Could you check a few things on this drawing? It's one solid part, dimensions in mm from its lowest x, y, z. Give positions to 0.01 mm unless a question says otherwise; leave off trailing zeros. Order: outer loops, then holes, each group sorted by start corner. A loop starts at its lowest first (then second) coordinate and runs counter-clockwise, first axis right, second up. Notation, with made-up numbers: M -16.5,40 L -4.5,40 A18 ccw -4.5,67 Z; hole C 4,22.5 d5. An arc over 180 degrees is marked long. Use CSV: the item, a comma, the result in double quotes. Start each with the question number.
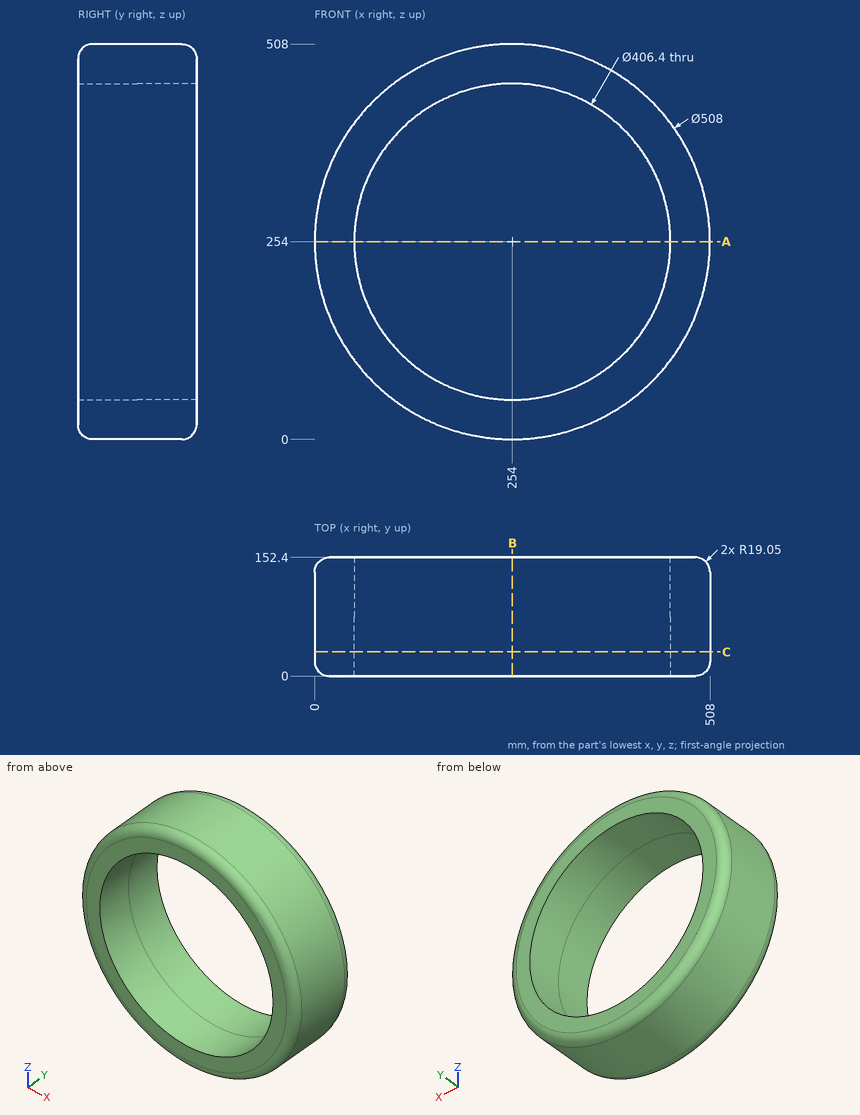
Q1. For P1, Ø1.5, axis at x = 429.5, y = 68, coming from the -Z side; P2, Ø12, axis at x = 357, y = 104.5, coming from the +Z side; P3, Ø4, axis at x = 139, y = 33.5, coming from the +Z side, each with a flat end and sliding along its axis, tell me the tip position at first contact or that it passes through.
Q2. Imagine slicing it at A-A, the plane z = 254. Please give me the cut outline in (x, y), then the cut area to 3 significant figures.
Q3. I need wall thicknesses on line 1 (Z direction, x = 254, y = 17); line 2 (Z direction, x = 255, y = 75.5); line 3 (X direction, y = 88.5, z = 110.5). Which ranges of each line are inside material? Lowest first, please. Write a range as [from, to].
Q4. Imagine slicing it at C-C, the plane y = 31. Please give me the cut outline in (x, z), then the cut area to 3 significant figures.
Q5. Imagine slicing it at B-B, the plane x = 254. Please give me the cut outline in (y, z), then the cut area to 3 significant figures.
Reply:
1,P1,"stops at z = 69.67"
1,P2,"stops at z = 488.75"
1,P3,"stops at z = 481.48"
2,outline,"M 0,19.05 A19.05 ccw 19.05,0 L 50.8,0 L 50.8,152.4 L 19.05,152.4 A19.05 ccw 0,133.35 Z; M 457.2,0 L 488.95,0 A19.05 ccw 508,19.05 L 508,133.35 A19.05 ccw 488.95,152.4 L 457.2,152.4 Z"
2,area,"15,200 mm^2"
3,line 1,"z = [0.11, 50.8], [457.2, 507.89]"
3,line 2,"z = [0, 50.8], [457.2, 508]"
3,line 3,"x = [44.42, 110.13], [397.87, 463.58]"
4,outline,"C 254,254 d508; hole C 254,254 d406.4"
4,area,"73,000 mm^2"
5,outline,"M 0,19.05 A19.05 ccw 19.05,0 L 133.35,0 A19.05 ccw 152.4,19.05 L 152.4,50.8 L 0,50.8 Z; M 0,457.2 L 152.4,457.2 L 152.4,488.95 A19.05 ccw 133.35,508 L 19.05,508 A19.05 ccw 0,488.95 Z"
5,area,"15,200 mm^2"
